Part model, mm, in its own coordinate system. Give positions to 0.01 mm unless a question says otherwise; leave off trailing zeros. Order: outer loops, then holes, each group sorted by start corner. A loop starts at its lowest first (then second) coordinate and runs counter-clockwise, first axis right, second up. Notation, with made-up numbers: M 78,71 L 100,71 A33 ccw 100,106 Z; hole C 75.5,-15 d9. An arc over 180 degrees is marked long. Return JSON: item names as keys, results as strings.
Autodesk Inventor part; units mm, degrees
ref_plane "XY Plane" through (0, 0, 0) normal (0, 0, 1) x (1, 0, 0)
sketch "Sketch1" plane through (0, 0, 0) normal (0, 0, 1) x (1, 0, 0)
  line L0 (41, -67.75) -> (-41, -67.75)
  line L1 (-41, -67.75) -> (-41, 67.75)
  line L2 (-41, 67.75) -> (41, 67.75)
  line L3 (41, 67.75) -> (41, -67.75)
  line L4 (41, -67.75) -> (-41, 67.75) construction
  line L5 (-41, -67.75) -> (41, 67.75) construction
  circle A0 centre (0, 0) radius 12.75
  line L6 (11.3137, -11.3137) -> (-11.3137, -11.3137) construction
  line L7 (-11.3137, -11.3137) -> (-11.3137, 11.3137) construction
  line L8 (-11.3137, 11.3137) -> (11.3137, 11.3137) construction
  line L9 (11.3137, 11.3137) -> (11.3137, -11.3137) construction
  line L10 (11.3137, -11.3137) -> (-11.3137, 11.3137) construction
  line L11 (-11.3137, -11.3137) -> (11.3137, 11.3137) construction
  circle A1 centre (0, 0) radius 16 construction
  line L12 (0, 16) -> (0, -16) construction
  dimension "d0" = 82
  dimension "d1" = 135.5
  dimension "d2" = 25.5
  dimension "d3" = 32
  dimension "d4" = 0
extrude "Extrusion1" add sketch "Sketch1" along normal blind 6.35
hole "Hole1" at (0, 16, 0) at (11.3137, 11.3137, 0) at (-11.3137, 11.3137, 0) at (11.3137, -11.3137, 0) at (0, -16, 0) at (-11.3137, -11.3137, 0) direction (0, 0, 1) diameter 3.242 end through all
fillet "Fillet1" radius 2 4 edges at (41, 67.75, 3.175) (-41, 67.75, 3.175) (-41, -67.75, 3.175) (41, -67.75, 3.175)
sketch "Sketch2" plane through (0, 0, 6.35) normal (0, 0, 1) x (1, 0, 0)
  line L0 (32.5, -58) -> (-32.5, -58) construction
  line L1 (-32.5, -58) -> (-32.5, 58) construction
  line L2 (-32.5, 58) -> (32.5, 58) construction
  line L3 (32.5, 58) -> (32.5, -58) construction
  line L4 (32.5, -58) -> (-32.5, 58) construction
  line L5 (-32.5, -58) -> (32.5, 58) construction
  point P0 (0, 0)
  point P1 (32.5, 0)
  point P2 (-32.5, 0)
  dimension "d15" = 65
  dimension "d16" = 116
hole "Hole2" at (-32.5, 58, 6.35) at (32.5, 58, 6.35) at (32.5, 0, 6.35) at (32.5, -58, 6.35) at (-32.5, -58, 6.35) at (-32.5, 0, 6.35) direction (0, 0, -1) diameter 5.3 end through all
properties part number "Z-Axis Nut Plate" material "Aluminum 6061"
Q1. Band-saw the part on D-D (z = 2.5). Give the number of separate pieces and of enclosed holes in the cut face, then the cut area to 3 significant figures.
Established:
{"separate pieces": "1", "enclosed holes": "13", "area": "10,400 mm²"}
Q2. Two-plate mould, pull along Y, no slides. Class faces 1 (the flat face through (-1, 67.75, 3)), 2 (the flat face through (1, -67.75, 3)), 3 (the cylindrical face through (0.621, -14.503, 3.219)): +Y half, -Y half, draft (parallel to the pull), parting line (faces both ways), or undercut.
Established:
{"face 1": "+Y half", "face 2": "-Y half", "face 3": "undercut"}
Q3. Band-saw the part on A-A (y = 0). Give the cut face in (x, z).
Established:
{"outline": "M -41,0 L -35.15,0 L -35.15,6.35 L -41,6.35 Z; M -29.85,0 L -12.75,0 L -12.75,6.35 L -29.85,6.35 Z; M 12.75,0 L 29.85,0 L 29.85,6.35 L 12.75,6.35 Z; M 35.15,0 L 41,0 L 41,6.35 L 35.15,6.35 Z"}
Q4. Probe line 1 along Y through (x, z) = (0, 5); line 2 along Y through (x, z) = (32.5, 4.5); line 3 along X through (y, z) = (-15.5, 1.25). List the from-to ranges inside material, lowest first.
Established:
{"line 1": "y = -67.75 to -17.62, -14.38 to -12.75, 12.75 to 14.38, 17.62 to 67.75", "line 2": "y = -67.75 to -60.65, -55.35 to -2.65, 2.65 to 55.35, 60.65 to 67.75", "line 3": "x = -41 to -1.54, 1.54 to 41"}
Q5. Band-saw the part on C-C (y = 58). Give the cut face in (x, z).
Established:
{"outline": "M -41,0 L -35.15,0 L -35.15,6.35 L -41,6.35 Z; M -29.85,0 L 29.85,0 L 29.85,6.35 L -29.85,6.35 Z; M 35.15,0 L 41,0 L 41,6.35 L 35.15,6.35 Z"}
Q6. Band-saw the part on B-B (x = 32.5). Give the cut face in (y, z).
Established:
{"outline": "M -67.75,0 L -60.65,0 L -60.65,6.35 L -67.75,6.35 Z; M -55.35,0 L -2.65,0 L -2.65,6.35 L -55.35,6.35 Z; M 2.65,0 L 55.35,0 L 55.35,6.35 L 2.65,6.35 Z; M 60.65,0 L 67.75,0 L 67.75,6.35 L 60.65,6.35 Z"}
Q7. Pin check, flat tip, straight feed: pin 1 (4 mm diameter, centred on x = 11.31, y = -11.31, fed in from +Z). Stop position of the tip, or through.
Established:
{"pin 1": "stops at z = 6.35"}
